Work out the finished part from the listing and answer in its coordinate system (mm). A direction names the side the tool comes from. Round coordinates to 2 decimals unless told otherwise and drop trailing zeros. Order: outer loops, then holes, each group sorted by start corner. A loop starts at its lowest first (then second) coordinate and runs counter-clockwise, first axis right, second up. Notation, with made-up numbers: (7, 5) - (65, 5) arc R18 cw to (65, 14) - close; hole circle Ø1 at (83.5, -18). An arc over 180 degrees is marked (long way). Use one line per item in the form item = value. Start each with the question number.
Q1. Given P1, Ø5.5, axis at y = -12.01, z = 9.11, coming from the -X side; P2, Ø3, axis at y = -33.07, z = -8.57, coming from the -X side; P3, Ø7.5, axis at x = 22, z = -2, coming from the -Y side, each flat-ended and moving along its own axis, determine where each tip first touches the part or whether it passes through.
Q2. For a pull along Z with two mould halves and no side action, classify faces 3 (the flat face through (-6.35, -1, 0)), 4 (the cylindrical face through (37.295, -20.254, 3.286)), 5 (the flat face through (27, -1, -12.7)), 6 (the cylindrical face through (37.295, -31.405, -8.042)) as +Z half, -Z half, draft (parallel to the pull), parting line (faces both ways), or undercut.
Q3. The part is cut by section A-A on x = 0. Determine the outline of the cut face in (y, z).
Q4. Find the intervals of material crossed by line 1 (X direction, y = -16, z = 12); line 2 (Y direction, x = 20.5, z = 2.5); line 3 (X direction, y = -0.9, z = 0), in increasing order. Write a range as [from, to].
Q5. The part is cut by section B-B on y = -29.5. Determine the outline of the cut face in (x, z).
Q6. Which of the six approach directions +Z, -Z, +X, -X, +Y, -Y give full straight-line access (tool end or side, diameter ignored) to faces 1 (the flat face through (36.512, -22, -1)), 2 (the flat face through (37, -40.344, -1))?
Q7. The part is cut by section C-C on z = 0. Determine the outline of the cut face in (x, y).
from build123d import *

# Parameters (mm, degrees)
SKETCH1_R                    = 2.25
SKETCH1_R_2                  = 8
SKETCH1_R_3                  = 1.75
BASE_FLANGE1_DEPTH           = 1.5875
SKETCHED_START               = 38.1
SKETCHED_BEND1_OUTLINE_W     = 1.5875
SKETCHED_BEND1_OUTLINE_H     = 25.4
SKETCHED_BEND1_DEPTH         = 38.1
SKETCHED_START_2             = 36.5125
SKETCHED_BEND1_2_OUTLINE_R   = 1.75
SKETCHED_BEND1_2_OUTLINE_R_2 = 8
SKETCHED_BEND1_2_DEPTH       = 1.361458034
SKETCHED_START_3             = 35.7759
SKETCHED_BEND1_3_OUTLINE_R   = 1.75
SKETCHED_BEND1_3_OUTLINE_R_2 = 8
SKETCHED_BEND1_3_DEPTH       = 2.3241
SKETCHED_START_4             = -12.7
SKETCHED_BEND1_4_DEPTH       = 31.75
SKETCHED_START_5             = -1.5875
SKETCHED_BEND1_5_DEPTH       = 1.5875


with BuildPart() as part:
    # Base-Flange1: sheet metal written as solids
    # Sketch1 → Base-Flange1 (new body)
    with BuildSketch(Plane(origin=(0, 0, 0), x_dir=(1, 0, 0), z_dir=(0, 1, 0))):
        with BuildLine():
            Line((-3.175, 12.7), (38.1, 12.7))
            Line((38.1, 12.7), (73.025, 12.7))
            ThreePointArc((73.025, 12.7), (75.27006403, 11.77006403), (76.2, 9.525))
            Line((76.2, 9.525), (76.2, -6.35))
            ThreePointArc((76.2, -6.35), (68.03164054, -18.213988959), (54.033978895, -14.816666667))
            ThreePointArc((54.033978895, -14.816666667), (51.893344987, -13.2532696), (49.300968343, -12.7))
            Line((49.300968343, -12.7), (38.1, -12.7))
            Line((38.1, -12.7), (-3.175, -12.7))
            ThreePointArc((-3.175, -12.7), (-5.42006403, -11.77006403), (-6.35, -9.525))
            Line((-6.35, -9.525), (-6.35, 9.525))
            ThreePointArc((-6.35, 9.525), (-5.42006403, 11.77006403), (-3.175, 12.7))
        make_face()
        with Locations(Location((0, 0, 0), (0, 0, 270))):
            Circle(SKETCH1_R, mode=Mode.SUBTRACT)
        with Locations(Location((63.5, -6.35, 0), (0, 0, 270))):
            Circle(SKETCH1_R_2, mode=Mode.SUBTRACT)
        with Locations(Location((47.866176921, -9.10666482, 0), (0, 0, 270))):
            Circle(SKETCH1_R_3, mode=Mode.SUBTRACT)
        with Locations(Location((53.295746696, 5.810955535, 0), (0, 0, 270))):
            Circle(SKETCH1_R_3, mode=Mode.SUBTRACT)
        with Locations(Location((68.929569775, 8.567620355, 0), (0, 0, 270))):
            Circle(SKETCH1_R_3, mode=Mode.SUBTRACT)
    extrude(amount=-BASE_FLANGE1_DEPTH)

    # Sketched Bend1: read off the stored shape, not the designer's step
    # Sketched Bend1 outline → Sketched Bend1 (cut)
    with BuildSketch(Plane.YZ.offset(SKETCHED_START)):
        with Locations((-0.79375, 0)):
            Rectangle(SKETCHED_BEND1_OUTLINE_W, SKETCHED_BEND1_OUTLINE_H)
    extrude(amount=SKETCHED_BEND1_DEPTH, mode=Mode.SUBTRACT)

    # Sketched Bend1 2 outline → Sketched Bend1 2 (add)
    with BuildSketch(Plane.YZ.offset(SKETCHED_START_2)):
        with BuildLine():
            Line((-1.5875, 12.7), (-13.445300184, 12.7))
            ThreePointArc((-13.445300184, 12.7), (-16.037676829, 13.2532696), (-18.178310737, 14.816666667))
            ThreePointArc((-18.178310737, 14.816666667), (-32.175972382, 18.213988959), (-40.344331841, 6.35))
            Line((-40.344331841, 6.35), (-40.344331841, -9.525))
            ThreePointArc((-40.344331841, -9.525), (-39.414395871, -11.77006403), (-37.169331841, -12.7))
            Line((-37.169331841, -12.7), (-1.5875, -12.7))
            Line((-1.5875, -12.7), (-1.5875, 12.7))
        make_face()
        with Locations((-33.073901617, -8.567620355)):
            Circle(SKETCHED_BEND1_2_OUTLINE_R, mode=Mode.SUBTRACT)
        with Locations((-17.440078538, -5.810955535)):
            Circle(SKETCHED_BEND1_2_OUTLINE_R, mode=Mode.SUBTRACT)
        with Locations((-27.644331841, 6.35)):
            Circle(SKETCHED_BEND1_2_OUTLINE_R_2, mode=Mode.SUBTRACT)
        with Locations((-12.010508762, 9.10666482)):
            Circle(SKETCHED_BEND1_2_OUTLINE_R, mode=Mode.SUBTRACT)
    extrude(amount=SKETCHED_BEND1_2_DEPTH)

    # Sketched Bend1 3 outline → Sketched Bend1 3 (add)
    with BuildSketch(Plane.YZ.offset(SKETCHED_START_3)):
        with BuildLine():
            Line((-1.5875, 12.7), (-13.445300184, 12.7))
            ThreePointArc((-13.445300184, 12.7), (-16.037676829, 13.2532696), (-18.178310737, 14.816666667))
            ThreePointArc((-18.178310737, 14.816666667), (-32.175972382, 18.213988959), (-40.344331841, 6.35))
            Line((-40.344331841, 6.35), (-40.344331841, -9.525))
            ThreePointArc((-40.344331841, -9.525), (-39.414395871, -11.77006403), (-37.169331841, -12.7))
            Line((-37.169331841, -12.7), (-1.5875, -12.7))
            Line((-1.5875, -12.7), (-1.5875, 12.7))
        make_face()
        with Locations((-33.073901617, -8.567620355)):
            Circle(SKETCHED_BEND1_3_OUTLINE_R, mode=Mode.SUBTRACT)
        with Locations((-17.440078538, -5.810955535)):
            Circle(SKETCHED_BEND1_3_OUTLINE_R, mode=Mode.SUBTRACT)
        with Locations((-27.644331841, 6.35)):
            Circle(SKETCHED_BEND1_3_OUTLINE_R_2, mode=Mode.SUBTRACT)
        with Locations((-12.010508762, 9.10666482)):
            Circle(SKETCHED_BEND1_3_OUTLINE_R, mode=Mode.SUBTRACT)
    extrude(amount=SKETCHED_BEND1_3_DEPTH)

    # Sketched Bend1 4 outline → Sketched Bend1 4 (cut)
    with BuildSketch(Plane.XY.offset(SKETCHED_START_4)):
        with BuildLine():
            ThreePointArc((35.7759, 0), (37.41928687, -0.68071313), (38.1, -2.3241))
            Line((38.1, -2.3241), (38.1, 0))
            Line((38.1, 0), (35.7759, 0))
        make_face()
        with BuildLine():
            Line((36.5125, -40.344331841), (36.5125, -2.3241))
            ThreePointArc((36.5125, -2.3241), (36.296754855, -1.803245145), (35.7759, -1.5875))
            Line((35.7759, -1.5875), (35.7759, -40.344331841))
            Line((35.7759, -40.344331841), (36.5125, -40.344331841))
        make_face()
    extrude(amount=SKETCHED_BEND1_4_DEPTH, mode=Mode.SUBTRACT)

    # Sketched Bend1 5 outline → Sketched Bend1 5 (cut)
    with BuildSketch(Plane(origin=(0, 0, 0), x_dir=(1, 0, 0), z_dir=(0, 1, 0)).offset(SKETCHED_START_5)):
        with BuildLine():
            ThreePointArc((49.300968343, -12.7), (51.893344987, -13.2532696), (54.033978895, -14.816666667))
            ThreePointArc((54.033978895, -14.816666667), (64.80660234, -18.982608215), (74.498522628, -12.7))
            Line((74.498522628, -12.7), (68.365953144, -12.7))
            ThreePointArc((68.365953144, -12.7), (63.5, -14.35), (58.634046856, -12.7))
            Line((58.634046856, -12.7), (49.300968343, -12.7))
        make_face()
    extrude(amount=SKETCHED_BEND1_5_DEPTH, mode=Mode.SUBTRACT)


solid = part.part
Found:
q1.P1 = 36.51
q1.P2 = through
q1.P3 = -1.59
q2.face_3 = draft
q2.face_4 = undercut
q2.face_5 = -Z half
q2.face_6 = undercut
q3.outline = (-1.59, -12.7) - (0, -12.7) - (0, -2.25) - (-1.59, -2.25) - close; (-1.59, 2.25) - (0, 2.25) - (0, 12.7) - (-1.59, 12.7) - close
q4.line_1 = [36.51, 38.1]
q4.line_2 = [-1.59, 0]
q4.line_3 = [-6.35, -2.25], [2.25, 37.61]
q5.outline = (36.51, -12.7) - (38.1, -12.7) - (38.1, -1.43) - (36.51, -1.43) - close; (36.51, 14.13) - (38.1, 14.13) - (38.1, 18.91) - (36.51, 18.91) - close
q6.face_1 = +Z, -Z, -X, -Y
q6.face_2 = +Z, -Z, +X, -X, -Y
q7.outline = (-6.35, -1.59) - (-2.25, -1.59) - (-2.25, 0) - (-6.35, 0) - close; (2.25, -1.59) - (35.78, -1.59) arc R0.74 cw to (36.51, -2.32) - (36.51, -22.78) - (38.1, -22.78) - (38.1, -2.32) arc R2.32 ccw to (35.78, 0) - (2.25, 0) - close; (36.51, -40.34) - (38.1, -40.34) - (38.1, -32.51) - (36.51, -32.51) - close
